```python
from build123d import *

# Parameters (mm, degrees)
SKETCH1_W           = 24
SKETCH1_H           = 18
BOSS_EXTRUDE1_DEPTH = 5
SKETCH3_R           = 1.5575
CUT_EXTRUDE1_DEPTH  = 6
CUT_EXTRUDE2_DEPTH  = 6
SKETCH5_R           = 10
BOSS_EXTRUDE3_DEPTH = 2
SKETCH6_R           = 10
BOSS_EXTRUDE4_DEPTH = 2
SKETCH7_R           = 2
CUT_EXTRUDE3_DEPTH  = 29


with BuildPart() as part:
    # Sketch1 → Boss-Extrude1 (new body)
    with BuildSketch(Plane.XY):
        with Locations((12, -9)):
            Rectangle(SKETCH1_W, SKETCH1_H)
    extrude(amount=BOSS_EXTRUDE1_DEPTH)

    # Sketch3 → Cut-Extrude1 (cut, through all)
    with BuildSketch(Plane.XY.offset(5)):
        with Locations((3.59586, -15.22505)):
            Circle(SKETCH3_R)
        with Locations((19.14986, -15.22505)):
            Circle(SKETCH3_R)
    extrude(amount=-CUT_EXTRUDE1_DEPTH, mode=Mode.SUBTRACT)

    # Sketch4 → Cut-Extrude2 (cut, through all)
    with BuildSketch(Plane.XY.offset(5)):
        with BuildLine():
            Line((1.089474394, -2.489991356), (22.608748961, -2.489991356))
            ThreePointArc((22.608748961, -2.489991356), (23.368757605, -3.25), (22.608748961, -4.010008644))
            Line((22.608748961, -4.010008644), (1.089474394, -4.010008644))
            ThreePointArc((1.089474394, -4.010008644), (0.32946575, -3.25), (1.089474394, -2.489991356))
        make_face()
    extrude(amount=-CUT_EXTRUDE2_DEPTH, mode=Mode.SUBTRACT)

    # Sketch5 → Boss-Extrude3 (add)
    with BuildSketch(Plane.ZY):
        with Locations((2.5, -9)):
            Circle(SKETCH5_R)
    extrude(amount=BOSS_EXTRUDE3_DEPTH)

    # Sketch6 → Boss-Extrude4 (add)
    with BuildSketch(Plane(origin=(24, 0, 0), x_dir=(0, 0, -1), z_dir=(1, 0, 0))):
        with Locations((-2.5, -9)):
            Circle(SKETCH6_R)
    extrude(amount=BOSS_EXTRUDE4_DEPTH)

    # Sketch7 → Cut-Extrude3 (cut, through all)
    with BuildSketch(Plane(origin=(26, 0, 0), x_dir=(0, 0, -1), z_dir=(1, 0, 0))):
        with Locations((-2.5, -2.07616)):
            Circle(SKETCH7_R)
    extrude(amount=-CUT_EXTRUDE3_DEPTH, mode=Mode.SUBTRACT)


solid = part.part
```
Build history of the part. All positions in model axes, mm. A direction names the side the tool comes from. Round coordinates to 2 decimals unless told otherwise and drop trailing zeros. Order: outer loops, then holes, each group sorted by start corner. A loop starts at its lowest first (then second) coordinate and runs counter-clockwise, first axis right, second up. Notation, with made-up numbers: (86.25, 22.5) - (129.25, 22.5) arc R18 ccw to (129.25, 33.5) - close; hole circle Ø6 at (25.25, -22). An arc over 180 degrees is marked (long way). Use a Markdown table: item, result.
1) Saw through at D-D on z = 2.5. Write the cut outline in (x, y) (1 decimal), and give its area (3 significant figures).
Recorded:
| item | result |
|---|---|
| outline | (-2, -19) - (0, -19) - (0, -18) - (24, -18) - (24, -19) - (26, -19) - (26, -4.1) - (-2, -4.1) - close; (-2, -0.1) - (26, -0.1) - (26, 1) - (24, 1) - (24, 0) - (0, 0) - (0, 1) - (-2, 1) - close; hole circle Ø3.1 at (3.6, -15.2); hole circle Ø3.1 at (19.1, -15.2) |
| area | 385 mm² |
2) Saw through at C-C on y = -3.25. Write the cut outline in (x, z).
Recorded:
| item | result |
|---|---|
| outline | (-2, -5.68) - (0, -5.68) - (0, 0) - (0.33, 0) - (0.33, 0.88) - (-2, 0.88) - close; (-2, 4.12) - (0.33, 4.12) - (0.33, 5) - (0, 5) - (0, 10.68) - (-2, 10.68) - close; (23.37, 0) - (24, 0) - (24, -5.68) - (26, -5.68) - (26, 0.88) - (23.37, 0.88) - close; (23.37, 4.12) - (26, 4.12) - (26, 10.68) - (24, 10.68) - (24, 5) - (23.37, 5) - close |
3) Tool access for faces 1 (the face through (23.2, -3.73, 0.57)), 2 (the face through (12, -18, 2)), 3 (the face through (12, -9, 5)), 4 (the face through (11.8, 0, 1.9)), 5 (the face through (12, -9, 0)): list every direction of +Z, -Z, +X, -X, +Y, -Y with a clear straight run to the whole face (end or side of a thin tool).
Recorded:
| item | result |
|---|---|
| face 1 | +Z, -Z |
| face 2 | +Z, -Z, -Y |
| face 3 | +Z, +Y, -Y |
| face 4 | +Z, -Z, +Y |
| face 5 | -Z, +Y, -Y |
4) Pull direction X, two halves, no side cores. Call faces 6 (the face through (26, -9, 3)), 7 (the face through (12, -4.01, 1)), 8 (the face through (-0.99, -6, 12.04)): pulls with the +X half, pulls with the -X half, needs draft (parallel to the pull), parting line crosses it, or undercut.
Recorded:
| item | result |
|---|---|
| face 6 | pulls with the +X half |
| face 7 | undercut |
| face 8 | needs draft |
5) Saw through at A-A on z = 10.5. Write the cut outline in (x, y).
Recorded:
| item | result |
|---|---|
| outline | (-2, -15) - (0, -15) - (0, -3) - (-2, -3) - close; (24, -15) - (26, -15) - (26, -3) - (24, -3) - close |
6) Flat gauge pins, fed straight in: pin 1 Ø2 at (x, y) = (16, -7) entering from +Z; pin 2 Ø3.5 at (y, z) = (-2.08, 2.5) entering from +X; pin 3 Ø3 at (x, z) = (2, 0.5) entering from -Y; pin 4 Ø1 at (x, z) = (16.5, 4.5) entering from +Y. Where does each tip first touch, or does it go through?
Recorded:
| item | result |
|---|---|
| pin 1 | stops at z = 5 |
| pin 2 | passes through |
| pin 3 | stops at y = -18 |
| pin 4 | stops at y = 0 |
7) Wall check: L1, parallel to X at y = -14, z = 6.75; L2, parallel to Y at x = 18.25, z = 1; L3, parallel to Y at x = 0.5, z = 4.25. Give the ranges that are in metal, low to high.
Recorded:
| item | result |
|---|---|
| L1 | x = -2 to 0, 24 to 26 |
| L2 | y = -18 to -16.5, -13.95 to -4.01, -0.75 to 0 |
| L3 | y = -18 to -3.73, -1.11 to 0 |
8) Saw through at B-B on x = 12. Write the cut outline in (y, z).
Recorded:
| item | result |
|---|---|
| outline | (-18, 0) - (-4.01, 0) - (-4.01, 1.99) arc R2 cw to (-4.01, 3.01) - (-4.01, 5) - (-18, 5) - close; (-2.49, 0) - (0, 0) - (0, 5) - (-2.49, 5) - (-2.49, 4.46) arc R2 cw (long way) to (-2.49, 0.54) - close |
